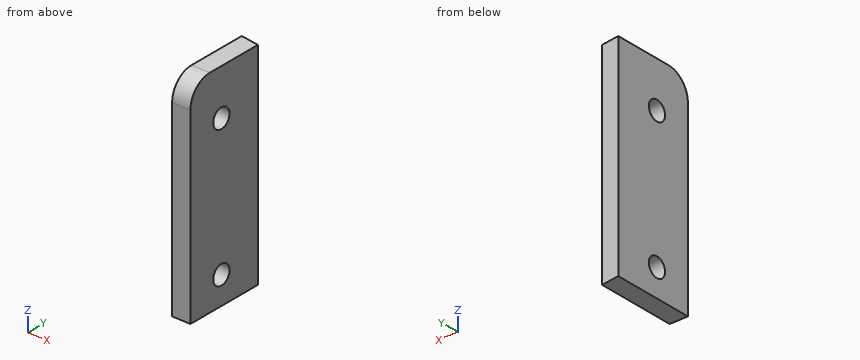
```python
from build123d import *

# Parameters (mm, degrees)
EXTRUSION1_DEPTH  = 46
CONG_1_R          = 5
TROU_TARAUD_M51_D = 4.2


with BuildPart() as part:
    # Esquisse1 → Extrusion1 (new body)
    with BuildSketch(Plane.XY):
        Polygon((0, 0), (4, 0), (4, 17.437836661), (0, 18), align=None)
    extrude(amount=EXTRUSION1_DEPTH)

    # Congé1
    cong_1_edges = [part.edges().sort_by_distance(p)[0] for p in [
        (2, 0, 46),
    ]]
    fillet(cong_1_edges, radius=CONG_1_R)

    # Trou taraudé M51 (through all)
    with Locations(Plane(origin=(4, 0, 0), x_dir=(0, 0, -1), z_dir=(1, 0, 0))):
        with Locations((-6, 8), (-36, 8)):
            Hole(TROU_TARAUD_M51_D / 2)


solid = part.part
```
Work out the finished part from the listing and answer in its coordinate system (mm). Round coordinates to 2 decimals unless told otherwise and drop trailing zeros. Order: outer loops, then holes, each group sorted by start corner. A loop starts at its lowest first (then second) coordinate and runs counter-clockwise, first axis right, second up.
Q1. Find the intervals of material crossed by line 1 along Z through (x, y) = (0.9, 7.25); line 2 along Z through (x, y) = (0.2, 6.25); line 3 along Y through (x, z) = (2.1, 6), in increasing order.
Solution:
line 1: z = 0 to 4.04, 7.96 to 34.04, 37.96 to 46
line 2: z = 0 to 4.84, 7.16 to 34.84, 37.16 to 46
line 3: y = 0 to 5.9, 10.1 to 17.7
Q2. A cutting plane is placed at B-B, the plane y = 8. Determine the outline of the cut face in (x, z), then the cut area to 3 significant figures.
Solution:
outline: (0, 0) - (4, 0) - (4, 3.9) - (0, 3.9) - close; (0, 8.1) - (4, 8.1) - (4, 33.9) - (0, 33.9) - close; (0, 38.1) - (4, 38.1) - (4, 46) - (0, 46) - close
area: 150 mm2
Q3. A cutting plane is placed at A-A, the plane z = 36. Determine the outline of the cut face in (x, y), then the cut area to 3 significant figures.
Solution:
outline: (0, 0) - (4, 0) - (4, 5.9) - (0, 5.9) - close; (0, 10.1) - (4, 10.1) - (4, 17.44) - (0, 18) - close
area: 54.1 mm2
Q4. Given pin 1 Ø1.5 at (x, z) = (1.5, 22.5) entering from +Y; pin 2 Ø2.5 at (y, z) = (8, 6) entering from +X; pin 3 Ø2 at (y, z) = (2, 20.5) entering from -X, each flat-ended and moving along its own axis, determine where each tip first touches the part or whether it passes through.
Solution:
pin 1: stops at y = 17.89
pin 2: passes through
pin 3: stops at x = 0
Q5. A cutting plane is placed at C-C, the plane x = 2.1. Determine the outline of the cut face in (y, z).
Solution:
outline: (0, 0) - (17.7, 0) - (17.7, 46) - (5, 46) arc R5 ccw to (0, 41) - close; hole circle Ø4.2 at (8, 6); hole circle Ø4.2 at (8, 36)
Q6. A cutting plane is placed at D-D, the plane y = 1. Determine the outline of the cut face in (x, z), then the cut area to 3 significant figures.
Solution:
outline: (0, 0) - (4, 0) - (4, 44) - (0, 44) - close
area: 176 mm2
